from build123d import *

# Parameters (mm, degrees)
SKETCH_1_W          = 70
SKETCH_1_H          = 70
EXTRUDE_1_DEPTH     = 5
SKETCH_2_R          = 8
CUT_EXTRUDE_1_DEPTH = 2.5
CUT_EXTRUDE_2_REACH = 4.5
SKETCH_3_R          = 6.5
SKETCH_4_W          = 70
SKETCH_4_H          = 70
SKETCH_4_R          = 10
CUT_EXTRUDE_3_DEPTH = 0.5
CUT_EXTRUDE_4_REACH = 7
SKETCH_5_R          = 1.6
CUT_EXTRUDE_6_REACH = 6.5
CUT_EXTRUDE_7_REACH = 6.5
FILLET_1_R          = 10
SKETCH_8_R          = 10
CUT_EXTRUDE_8_DEPTH = 0.5
EXTRUDE_2_DEPTH     = 4.5
CUT_EXTRUDE_9_REACH = 4
SKETCH_10_R         = 8
SKETCH_10_R_2       = 6.5


with BuildPart() as part:
    # 草图1 → 凸台-拉伸1 (new body)
    with BuildSketch(Plane(origin=(0, 0, 0), x_dir=(1, 0, 0), z_dir=(0, 1, 0))):
        Rectangle(SKETCH_1_W, SKETCH_1_H)
    extrude(amount=EXTRUDE_1_DEPTH)

    # 草图2 → 切除-拉伸1 (cut)
    with BuildSketch(Plane(origin=(0, 5, 0), x_dir=(1, 0, 0), z_dir=(0, 1, 0))):
        Circle(SKETCH_2_R)
    extrude(amount=-CUT_EXTRUDE_1_DEPTH, mode=Mode.SUBTRACT)

    # 草图3 → 切除-拉伸2 (cut, up to next)
    with BuildSketch(Plane(origin=(0, 2.5, 0), x_dir=(1, 0, 0), z_dir=(0, 1, 0)), mode=Mode.PRIVATE) as cut_extrude_2_sk1:
        Circle(SKETCH_3_R)
    cut_extrude_2_tool1 = extrude(cut_extrude_2_sk1.sketch, amount=-CUT_EXTRUDE_2_REACH, mode=Mode.PRIVATE) & part.part
    add(cut_extrude_2_tool1.solids().sort_by_distance((0, 2.5, 0))[0], mode=Mode.SUBTRACT)

    # 草图4 → 切除-拉伸3 (cut)
    with BuildSketch(Plane.XZ):
        Rectangle(SKETCH_4_W, SKETCH_4_H)
        Circle(SKETCH_4_R, mode=Mode.SUBTRACT)
    extrude(amount=-CUT_EXTRUDE_3_DEPTH, mode=Mode.SUBTRACT)

    # 草图5 → 切除-拉伸4 (cut, up to next)
    with BuildSketch(Plane(origin=(0, 5, 0), x_dir=(1, 0, 0), z_dir=(0, 1, 0)), mode=Mode.PRIVATE) as cut_extrude_4_sk1:
        with Locations((28.284271247, -28.284271247)):
            Circle(SKETCH_5_R)
    cut_extrude_4_tool1 = extrude(cut_extrude_4_sk1.sketch, amount=-CUT_EXTRUDE_4_REACH, mode=Mode.PRIVATE) & part.part
    add(cut_extrude_4_tool1.solids().sort_by_distance((28.284271, 5, 28.284271))[0], mode=Mode.SUBTRACT)
    # 草图5 → 切除-拉伸4 (cut, up to next)
    with BuildSketch(Plane(origin=(0, 5, 0), x_dir=(1, 0, 0), z_dir=(0, 1, 0)), mode=Mode.PRIVATE) as cut_extrude_4_sk2:
        with Locations((-28.284271247, -28.284271247)):
            Circle(SKETCH_5_R)
    cut_extrude_4_tool2 = extrude(cut_extrude_4_sk2.sketch, amount=-CUT_EXTRUDE_4_REACH, mode=Mode.PRIVATE) & part.part
    add(cut_extrude_4_tool2.solids().sort_by_distance((-28.284271, 5, 28.284271))[0], mode=Mode.SUBTRACT)
    # 草图5 → 切除-拉伸4 (cut, up to next)
    with BuildSketch(Plane(origin=(0, 5, 0), x_dir=(1, 0, 0), z_dir=(0, 1, 0)), mode=Mode.PRIVATE) as cut_extrude_4_sk3:
        with Locations((-28.284271247, 28.284271247)):
            Circle(SKETCH_5_R)
    cut_extrude_4_tool3 = extrude(cut_extrude_4_sk3.sketch, amount=-CUT_EXTRUDE_4_REACH, mode=Mode.PRIVATE) & part.part
    add(cut_extrude_4_tool3.solids().sort_by_distance((-28.284271, 5, -28.284271))[0], mode=Mode.SUBTRACT)
    # 草图5 → 切除-拉伸4 (cut, up to next)
    with BuildSketch(Plane(origin=(0, 5, 0), x_dir=(1, 0, 0), z_dir=(0, 1, 0)), mode=Mode.PRIVATE) as cut_extrude_4_sk4:
        with Locations((28.284271247, 28.284271247)):
            Circle(SKETCH_5_R)
    cut_extrude_4_tool4 = extrude(cut_extrude_4_sk4.sketch, amount=-CUT_EXTRUDE_4_REACH, mode=Mode.PRIVATE) & part.part
    add(cut_extrude_4_tool4.solids().sort_by_distance((28.284271, 5, -28.284271))[0], mode=Mode.SUBTRACT)

    # 草图6 → 切除-拉伸6 (cut, up to next)
    with BuildSketch(Plane.XZ.offset(-0.5), mode=Mode.PRIVATE) as cut_extrude_6_sk1:
        with BuildLine():
            Line((27.928932188, 35), (4.565391967, 11.636459779))
            ThreePointArc((4.565391967, 11.636459779), (0, 12.5), (-4.565391967, 11.636459779))
            Line((-4.565391967, 11.636459779), (-27.928932188, 35))
            Line((-27.928932188, 35), (27.928932188, 35))
        make_face()
    cut_extrude_6_tool1 = extrude(cut_extrude_6_sk1.sketch, amount=-CUT_EXTRUDE_6_REACH, mode=Mode.PRIVATE) & part.part
    add(cut_extrude_6_tool1.solids().sort_by_distance((0, 0.5, 26.217235))[0], mode=Mode.SUBTRACT)
    # 草图6 → 切除-拉伸6 (cut, up to next)
    with BuildSketch(Plane.XZ.offset(-0.5), mode=Mode.PRIVATE) as cut_extrude_6_sk2:
        with BuildLine():
            Line((35, -27.928932188), (11.636459779, -4.565391967))
            ThreePointArc((11.636459779, -4.565391967), (12.5, 0), (11.636459779, 4.565391967))
            Line((11.636459779, 4.565391967), (35, 27.928932188))
            Line((35, 27.928932188), (35, -27.928932188))
        make_face()
    cut_extrude_6_tool2 = extrude(cut_extrude_6_sk2.sketch, amount=-CUT_EXTRUDE_6_REACH, mode=Mode.PRIVATE) & part.part
    add(cut_extrude_6_tool2.solids().sort_by_distance((26.217235, 0.5, 0))[0], mode=Mode.SUBTRACT)
    # 草图6 → 切除-拉伸6 (cut, up to next)
    with BuildSketch(Plane.XZ.offset(-0.5), mode=Mode.PRIVATE) as cut_extrude_6_sk3:
        with BuildLine():
            Line((-27.928932188, -35), (-4.565391967, -11.636459779))
            ThreePointArc((-4.565391967, -11.636459779), (0, -12.5), (4.565391967, -11.636459779))
            Line((4.565391967, -11.636459779), (27.928932188, -35))
            Line((27.928932188, -35), (-27.928932188, -35))
        make_face()
    cut_extrude_6_tool3 = extrude(cut_extrude_6_sk3.sketch, amount=-CUT_EXTRUDE_6_REACH, mode=Mode.PRIVATE) & part.part
    add(cut_extrude_6_tool3.solids().sort_by_distance((0, 0.5, -26.217235))[0], mode=Mode.SUBTRACT)
    # 草图6 → 切除-拉伸6 (cut, up to next)
    with BuildSketch(Plane.XZ.offset(-0.5), mode=Mode.PRIVATE) as cut_extrude_6_sk4:
        with BuildLine():
            Line((-35, 27.928932188), (-11.636459779, 4.565391967))
            ThreePointArc((-11.636459779, 4.565391967), (-12.5, 0), (-11.636459779, -4.565391967))
            Line((-11.636459779, -4.565391967), (-35, -27.928932188))
            Line((-35, -27.928932188), (-35, 27.928932188))
        make_face()
    cut_extrude_6_tool4 = extrude(cut_extrude_6_sk4.sketch, amount=-CUT_EXTRUDE_6_REACH, mode=Mode.PRIVATE) & part.part
    add(cut_extrude_6_tool4.solids().sort_by_distance((-26.217235, 0.5, 0))[0], mode=Mode.SUBTRACT)

    # 草图7 → 切除-拉伸7 (cut, up to next)
    with BuildSketch(Plane.XZ.offset(-0.5), mode=Mode.PRIVATE) as cut_extrude_7_sk1:
        with BuildLine():
            Line((35, 27.928932188), (35, 35))
            Line((35, 35), (27.928932188, 35))
            Line((27.928932188, 35), (24.748737342, 31.819805153))
            ThreePointArc((24.748737342, 31.819805153), (31.819805153, 31.819805153), (31.819805153, 24.748737342))
            Line((31.819805153, 24.748737342), (35, 27.928932188))
        make_face()
    cut_extrude_7_tool1 = extrude(cut_extrude_7_sk1.sketch, amount=-CUT_EXTRUDE_7_REACH, mode=Mode.PRIVATE) & part.part
    add(cut_extrude_7_tool1.solids().sort_by_distance((32.243136, 0.5, 32.243136))[0], mode=Mode.SUBTRACT)
    # 草图7 → 切除-拉伸7 (cut, up to next)
    with BuildSketch(Plane.XZ.offset(-0.5), mode=Mode.PRIVATE) as cut_extrude_7_sk2:
        with BuildLine():
            Line((27.928932188, -35), (24.748737342, -31.819805153))
            ThreePointArc((24.748737342, -31.819805153), (31.819805153, -31.819805153), (31.819805153, -24.748737342))
            Line((31.819805153, -24.748737342), (35, -27.928932188))
            Line((35, -27.928932188), (35, -35))
            Line((35, -35), (27.928932188, -35))
        make_face()
    cut_extrude_7_tool2 = extrude(cut_extrude_7_sk2.sketch, amount=-CUT_EXTRUDE_7_REACH, mode=Mode.PRIVATE) & part.part
    add(cut_extrude_7_tool2.solids().sort_by_distance((32.243136, 0.5, -32.243136))[0], mode=Mode.SUBTRACT)
    # 草图7 → 切除-拉伸7 (cut, up to next)
    with BuildSketch(Plane.XZ.offset(-0.5), mode=Mode.PRIVATE) as cut_extrude_7_sk3:
        with BuildLine():
            Line((-35, -27.928932188), (-31.819805153, -24.748737342))
            ThreePointArc((-31.819805153, -24.748737342), (-31.819805153, -31.819805153), (-24.748737342, -31.819805153))
            Line((-24.748737342, -31.819805153), (-27.928932188, -35))
            Line((-27.928932188, -35), (-35, -35))
            Line((-35, -35), (-35, -27.928932188))
        make_face()
    cut_extrude_7_tool3 = extrude(cut_extrude_7_sk3.sketch, amount=-CUT_EXTRUDE_7_REACH, mode=Mode.PRIVATE) & part.part
    add(cut_extrude_7_tool3.solids().sort_by_distance((-32.243136, 0.5, -32.243136))[0], mode=Mode.SUBTRACT)
    # 草图7 → 切除-拉伸7 (cut, up to next)
    with BuildSketch(Plane.XZ.offset(-0.5), mode=Mode.PRIVATE) as cut_extrude_7_sk4:
        with BuildLine():
            Line((-27.928932188, 35), (-24.748737342, 31.819805153))
            ThreePointArc((-24.748737342, 31.819805153), (-31.819805153, 31.819805153), (-31.819805153, 24.748737342))
            Line((-31.819805153, 24.748737342), (-35, 27.928932188))
            Line((-35, 27.928932188), (-35, 35))
            Line((-35, 35), (-27.928932188, 35))
        make_face()
    cut_extrude_7_tool4 = extrude(cut_extrude_7_sk4.sketch, amount=-CUT_EXTRUDE_7_REACH, mode=Mode.PRIVATE) & part.part
    add(cut_extrude_7_tool4.solids().sort_by_distance((-32.243136, 0.5, 32.243136))[0], mode=Mode.SUBTRACT)

    # 圆角1
    fillet_1_edges = [part.edges().sort_by_distance(p)[0] for p in [
        (4.565391967, 2.75, 11.636459779),
        (-4.565391967, 2.75, 11.636459779),
        (11.636459779, 2.75, -4.565391967),
        (11.636459779, 2.75, 4.565391967),
        (-4.565391967, 2.75, -11.636459779),
        (4.565391967, 2.75, -11.636459779),
        (-11.636459779, 2.75, 4.565391967),
        (-11.636459779, 2.75, -4.565391967),
    ]]
    fillet(fillet_1_edges, radius=FILLET_1_R)

    # 草图8 → 切除-拉伸8 (cut)
    with BuildSketch(Plane.XZ):
        Circle(SKETCH_8_R)
    extrude(amount=-CUT_EXTRUDE_8_DEPTH, mode=Mode.SUBTRACT)

    # 草图9 → 凸台-拉伸2 (add)
    with BuildSketch(Plane.XZ.offset(-0.5)):
        with BuildLine():
            Line((8.32300732, 15.394075132), (21.464466094, 28.535533906))
            ThreePointArc((21.464466094, 28.535533906), (0, 19.644660941), (-21.464466094, 28.535533906))
            Line((-21.464466094, 28.535533906), (-8.32300732, 15.394075132))
            ThreePointArc((-8.32300732, 15.394075132), (-4.820160406, 13.123419354), (-0.695521949, 12.480634969))
            ThreePointArc((-0.695521949, 12.480634969), (0, 12.5), (0.695521949, 12.480634969))
            ThreePointArc((0.695521949, 12.480634969), (4.820160406, 13.123419354), (8.32300732, 15.394075132))
        make_face()
        with BuildLine():
            Line((28.535533906, 21.464466094), (15.394075132, 8.32300732))
            ThreePointArc((15.394075132, 8.32300732), (13.123419354, 4.820160406), (12.480634969, 0.695521949))
            ThreePointArc((12.480634969, 0.695521949), (12.5, 0), (12.480634969, -0.695521949))
            ThreePointArc((12.480634969, -0.695521949), (13.123419354, -4.820160406), (15.394075132, -8.32300732))
            Line((15.394075132, -8.32300732), (28.535533906, -21.464466094))
            ThreePointArc((28.535533906, -21.464466094), (19.644660941, 0), (28.535533906, 21.464466094))
        make_face()
        with BuildLine():
            Line((21.464466094, -28.535533906), (8.32300732, -15.394075132))
            ThreePointArc((8.32300732, -15.394075132), (4.820160406, -13.123419354), (0.695521949, -12.480634969))
            ThreePointArc((0.695521949, -12.480634969), (0, -12.5), (-0.695521949, -12.480634969))
            ThreePointArc((-0.695521949, -12.480634969), (-4.820160406, -13.123419354), (-8.32300732, -15.394075132))
            Line((-8.32300732, -15.394075132), (-21.464466094, -28.535533906))
            ThreePointArc((-21.464466094, -28.535533906), (0, -19.644660941), (21.464466094, -28.535533906))
        make_face()
        with BuildLine():
            Line((-28.535533906, -21.464466094), (-15.394075132, -8.32300732))
            ThreePointArc((-15.394075132, -8.32300732), (-13.123419354, -4.820160406), (-12.480634969, -0.695521949))
            ThreePointArc((-12.480634969, -0.695521949), (-12.5, 0), (-12.480634969, 0.695521949))
            ThreePointArc((-12.480634969, 0.695521949), (-13.123419354, 4.820160406), (-15.394075132, 8.32300732))
            Line((-15.394075132, 8.32300732), (-28.535533906, 21.464466094))
            ThreePointArc((-28.535533906, 21.464466094), (-19.644660941, 0), (-28.535533906, -21.464466094))
        make_face()
    extrude(amount=-EXTRUDE_2_DEPTH)

    # 草图10 → 切除-拉伸9 (cut, up to next)
    with BuildSketch(Plane(origin=(0, 2.5, 0), x_dir=(1, 0, 0), z_dir=(0, 1, 0)), mode=Mode.PRIVATE) as cut_extrude_9_sk1:
        Circle(SKETCH_10_R)
        Circle(SKETCH_10_R_2, mode=Mode.SUBTRACT)
    cut_extrude_9_tool1 = extrude(cut_extrude_9_sk1.sketch, amount=-CUT_EXTRUDE_9_REACH, mode=Mode.PRIVATE) & part.part
    add(cut_extrude_9_tool1.solids().sort_by_distance((-7.773726, 2.5, 0))[0], mode=Mode.SUBTRACT)


solid = part.part
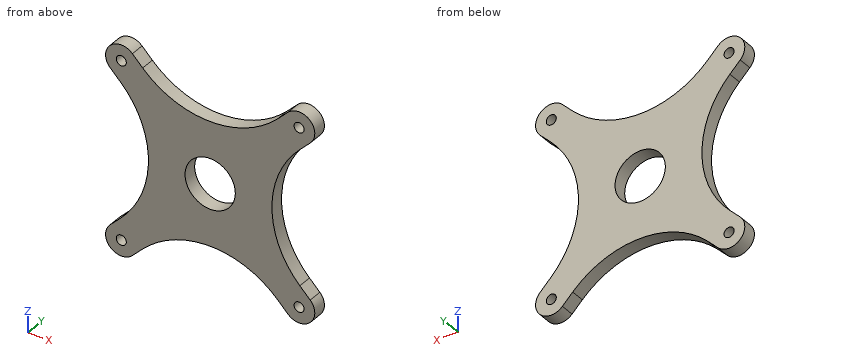
Check sheet for the modelled part. Datum: model origin and axes. Units: mm. Round coordinates to 2 decimals unless told otherwise and drop trailing zeros. Order: outer loops, then holes, each group sorted by start corner. A loop starts at its lowest first (then second) coordinate and runs counter-clockwise, first axis right, second up.
Q1. Cross-section at A-A, the plane z = 0. Enter the section's corners in (x, y), plus the area to 3 significant figures.
Filled sheet:
outline: (-19.64, 0.5) - (-8, 0.5) - (-8, 5) - (-19.64, 5) - close; (8, 0.5) - (19.64, 0.5) - (19.64, 5) - (8, 5) - close
area: 105 mm2
Q2. Cross-section at D-D, the plane z = 15. Enter the section's corners in (x, y).
Filled sheet:
outline: (-23.61, 0.5) - (23.61, 0.5) - (23.61, 5) - (-23.61, 5) - close
Q3. Depth check by flat-ended pin: P1, Ø1, axis at x = 14, y = 2.5, coming from the -Z side; P2, Ø2, axis at y = 1, z = 1.5, coming from the +X side; P3, Ø2, axis at y = 1.5, z = -24, coming from the -X side. Enter the tip coordinate at first touch or a pass-through.
Filled sheet:
P1: stops at z = -23.33
P2: stops at x = 19.75
P3: stops at x = -32.05
Q4. Scan lines: L1, parallel to Z at x = 0, y = 4; L2, parallel to X at y = 4.4, z = -29.5. Record each from-to range of solid material in increasing order.
Filled sheet:
L1: z = -19.64 to -8, 8 to 19.64
L2: x = -33.13 to -29.32, -27.24 to -22.43, 22.43 to 27.24, 29.32 to 33.13
Q5. Cross-section at C-C, the plane y = 1.35. Enter the section's corners in (x, z), plus the area to 3 significant figures.
Filled sheet:
outline: (-31.82, -24.75) arc R5 ccw to (-24.75, -31.82) - (-21.46, -28.54) arc R30.36 cw to (21.46, -28.54) - (24.75, -31.82) arc R5 ccw to (31.82, -24.75) - (28.54, -21.46) arc R30.36 cw to (28.54, 21.46) - (31.82, 24.75) arc R5 ccw to (24.75, 31.82) - (21.46, 28.54) arc R30.36 cw to (-21.46, 28.54) - (-24.75, 31.82) arc R5 ccw to (-31.82, 24.75) - (-28.54, 21.46) arc R30.36 cw to (-28.54, -21.46) - close; hole circle Ø3.2 at (-28.28, -28.28); hole circle Ø3.2 at (-28.28, 28.28); hole circle Ø16 at (0, 0); hole circle Ø3.2 at (28.28, -28.28); hole circle Ø3.2 at (28.28, 28.28)
area: 2,210 mm2
Q6. Cross-section at B-B, the plane x = -5.5. Enter the section's corners in (y, z), plus the area to 3 significant figures.
Filled sheet:
outline: (0.5, -20.15) - (5, -20.15) - (5, -5.81) - (0.5, -5.81) - close; (0.5, 5.81) - (5, 5.81) - (5, 20.15) - (0.5, 20.15) - close
area: 129 mm2
